Here's how the part is built. I have some questions about the finished solid (model axes, mm). A direction names the side the tool comes from. Round coordinates to 2 decimals unless told otherwise and drop trailing zeros. Loops run counter-clockwise (first coordinate to the right, second up) from the corner with the lowest first, then second, coordinate; pieces in that order, holes last. Notation, with made-up numbers: (-9.75, 26.25) - (15.25, 26.25) arc R31 cw to (15.25, 61.25) - close; hole circle Ø5 at (15.25, 73). An arc over 180 degrees is marked (long way). Answer as a JSON object with one key per item and string values. Group by question number.
1) Which directions (+Z, -Z, +X, -X, +Y, -Y) give clear straight access to the entire face, cutting with the end or side of a thin tool? Please do faces 1 (the face through (2, 0, 7)), 2 (the face through (9, 7.5, 2)).
2) I want a section at D-D, the plane y = 25.5. Please give me the cut outline in (x, z).
3) Will these pins go through, and if not, where does the flat tip stop? P1, Ø3, axis at y = 12.5, z = 9, coming from the -X side; P2, Ø4, axis at y = 30, z = 9, coming from the +X side; P3, Ø1.5, axis at x = 8.5, z = 2, coming from the -Y side; P4, Ø4.5, axis at x = 9, y = 22.5, coming from the +Z side.
4) I want a section at B-B, the plane y = 62.5. Please give me the cut outline in (x, z).
5) If I drill on line 1 along Z through (x, y) = (3, 12.5); line 2 along Y through (x, z) = (3.75, 9.5); line 3 along X through (y, z) = (15.5, 4.75), over which ranges is the centre line in solid material (lowest first)? Write a range as [from, to].
6) I want a section at A-A, the plane z = 9. Please give me the cut outline in (x, y).
7) I want a section at C-C, the plane z = 4. Please give me the cut outline in (x, y), then the cut area to 3 significant figures.
8) If we mould it in two halves opening along Y, with no side actions, what happens to faces 3 (the face through (11, 27, 5)), 4 (the face through (18.4, 9.5, 2.5)), 5 (the face through (2.465, 12.89, 7.243))? For each: pulls with the +Y half, pulls with the -Y half, needs draft (parallel to the pull), parting line crosses it, or undercut.
from build123d import *

# Parameters (mm, degrees)
F1_DEPTH = 14
F2_R     = 1.8
F3_DEPTH = 25
F4_DEPTH = 5


with BuildPart() as f1:
    # F0 (on Top) → F1 (new body)
    with BuildSketch(Plane.XY):
        Polygon((0, 68.5), (0, 0), (5, 0), (5, 7.5), (5, 21.5), (5, 56.5), (5, 68.5), align=None)
    extrude(amount=F1_DEPTH)

    # F2 (on face) → F3 (cut)
    with BuildSketch(Plane(origin=(0, 0, 0), x_dir=(0, -1, 0), z_dir=(-1, 0, 0))):
        with Locations((-62.5, 9)):
            Circle(F2_R)
        with Locations((-12.5, 9)):
            Circle(F2_R)
    extrude(amount=-F3_DEPTH, mode=Mode.SUBTRACT)

    # F0 (on Top) → F4 (join)
    with BuildSketch(Plane.XY):
        with BuildLine():
            Line((5, 56.5), (5, 21.5))
            Line((5, 21.5), (13.5, 21.5))
            ThreePointArc((13.5, 21.5), (17.472758, 20.263436), (20.041924, 16.990628))
            Line((20.041924, 16.990628), (5, 56.5))
        make_face()
        with BuildLine():
            Line((5, 21.5), (5, 7.5))
            Line((5, 7.5), (13.5, 7.5))
            ThreePointArc((13.5, 7.5), (6.5, 14.5), (13.5, 21.5))
            Line((13.5, 21.5), (5, 21.5))
        make_face()
        with BuildLine():
            Line((13.5, 12.25), (13.5, 7.5))
            ThreePointArc((13.5, 7.5), (18.449747, 9.550253), (20.5, 14.5))
            ThreePointArc((20.5, 14.5), (20.384529, 15.766201), (20.041924, 16.990628))
            ThreePointArc((20.041924, 16.990628), (17.472758, 20.263436), (13.5, 21.5))
            Line((13.5, 21.5), (13.5, 16.75))
            ThreePointArc((13.5, 16.75), (15.09099, 16.09099), (15.75, 14.5))
            ThreePointArc((15.75, 14.5), (15.09099, 12.90901), (13.5, 12.25))
        make_face()
        with BuildLine():
            ThreePointArc((13.5, 21.5), (6.5, 14.5), (13.5, 7.5))
            Line((13.5, 7.5), (13.5, 12.25))
            ThreePointArc((13.5, 12.25), (11.25, 14.5), (13.5, 16.75))
            Line((13.5, 16.75), (13.5, 21.5))
        make_face()
    extrude(amount=F4_DEPTH)


solid = f1.part
Outcome:
{
 "1": {"face 1": "+Z, -Z, +X, -X, -Y", "face 2": "+Z, -Z, +X, -Y"},
 "2": {"outline": "(0, 0) - (16.8, 0) - (16.8, 5) - (5, 5) - (5, 14) - (0, 14) - close"},
 "3": {"P1": "through", "P2": "x = 5", "P3": "y = 7.5", "P4": "z = 5"},
 "4": {"outline": "(0, 0) - (5, 0) - (5, 7.2) - (0, 7.2) - close; (0, 10.8) - (5, 10.8) - (5, 14) - (0, 14) - close"},
 "5": {"line 1": "[0, 7.2], [10.8, 14]", "line 2": "[0, 10.77], [14.23, 60.77], [64.23, 68.5]", "line 3": "[0, 11.48], [15.52, 20.43]"},
 "6": {"outline": "(0, 0) - (5, 0) - (5, 10.7) - (0, 10.7) - close; (0, 14.3) - (5, 14.3) - (5, 60.7) - (0, 60.7) - close; (0, 64.3) - (5, 64.3) - (5, 68.5) - (0, 68.5) - close"},
 "7": {"outline": "(0, 0) - (5, 0) - (5, 7.5) - (13.5, 7.5) arc R7 ccw to (20.5, 14.5) arc R7 ccw to (20.04, 16.99) - (5, 56.5) - (5, 68.5) - (0, 68.5) - close; hole circle Ø4.5 at (13.5, 14.5)", "area": "760 mm^2"},
 "8": {"face 3": "needs draft", "face 4": "pulls with the -Y half", "face 5": "undercut"}
}
